Part model, mm, in its own coordinate system. A direction names the side the tool comes from. Round coordinates to 2 decimals unless told otherwise and drop trailing zeros. Loops run counter-clockwise (first coordinate to the right, second up) from the corner with the lowest first, then second, coordinate; pieces in that order, holes last. Notation, with made-up numbers: (-4, 13) - (46, 13) arc R31 cw to (46, 45) - close; hole circle Ø2 at (12, 31.25). An arc over 180 degrees is marked (long way). Put each result on its own line as item: value.
from build123d import *

# Parameters (mm, degrees)
BOSS_EXTRUDE1_DEPTH = 13


with BuildPart() as part:
    # Sketch1 → Boss-Extrude1 (new body)
    with BuildSketch(Plane.XY):
        with BuildLine():
            Line((169.562304459, -46.160309931), (169.552568547, -34.320764913))
            ThreePointArc((169.552568547, -34.320764913), (167.950993273, -32.115534783), (165.631816979, -30.683925688))
            Line((165.631816979, -30.683925688), (164.32472896, -30.359173472))
            ThreePointArc((164.32472896, -30.359173472), (159.414987624, -30.865423823), (155.959571946, -34.389902778))
            Line((155.959571946, -34.389902778), (153.531390597, -39.695181294))
            Line((153.531390597, -39.695181294), (157.716593531, -42.649808935))
            ThreePointArc((157.716593531, -42.649808935), (158.460324124, -45.836019732), (155.520515025, -47.27219413))
            Line((155.520515025, -47.27219413), (152.052832095, -46.502518371))
            add(Edge.make_bspline(
                [(158.254307893, -49.702990605), (156.613856565, -49.334233495), (153.519768391, -49.291899755), (152.26174626, -47.033082798), (152.052832095, -46.502518371)],
                knots=[0, 0, 0, 0, 0.763192253, 1, 1, 1, 1], degree=3))
            Line((158.254307893, -49.702990605), (158.172150747, -49.796885596))
            Line((158.172150747, -49.796885596), (169.562304459, -46.160309931))
        make_face()
    extrude(amount=BOSS_EXTRUDE1_DEPTH)


solid = part.part
1. Band-saw the part on B-B (y = -44). List the corners of the cut face in (x, z).
A:
outline: (158.62, 0) - (169.56, 0) - (169.56, 13) - (158.62, 13) - close
2. Band-saw the part on A-A (x = 159). List the corners of the cut face in (y, z).
A:
outline: (-49.53, 0) - (-31.08, 0) - (-31.08, 13) - (-49.53, 13) - close
3. Pin check, flat tips, straight feed: P1, Ø5, axis at y = -34, z = 9.5, coming from the -X side; P2, Ø3, axis at x = 156.5, z = 2.5, coming from the -Y side; P3, Ø5, axis at y = -35.5, z = 4.5, coming from the -X side; P4, Ø2, axis at x = 156.5, y = -36.5, coming from the -Z side. Stop position of each tip, or through.
A:
P1: stops at x = 154.99
P2: stops at y = -49.65
P3: stops at x = 154.31
P4: stops at z = 0
4. Probe line 1 along Y through (x, z) = (155.25, 5.5); line 2 along Y through (x, z) = (155.5, 1.75); line 3 along X through (y, z) = (-42.75, 5.75). List the from-to ranges inside material, lowest first. Write a range as [from, to].
A:
line 1: y = [-49.14, -47.21], [-40.91, -35.94]
line 2: y = [-49.2, -47.27], [-41.08, -35.39]
line 3: x = [157.84, 169.56]
5. Two-plate mould, pull along X, no slides. Class faces 1 (the flat face through (163.8, -48, 6.4)), 2 (the flat face through (153.811, -46.893, 6.409)), 3 (the cylindrical face through (158.48, -45.79, 6.41)), 4 (the cylindrical face through (159.479, -30.835, 6.409)): pulls with the +X half, pulls with the -X half, needs draft (parallel to the pull), parting line crosses it, or undercut.
A:
face 1: pulls with the +X half
face 2: undercut
face 3: undercut
face 4: parting line crosses it
6. Tool access for faces 5 (the flat face through (154.76, -37.01, 6.41)), 6 (the flat face through (155.59, -41.15, 6.41)): list every direction of +Z, -Z, +X, -X, +Y, -Y with a clear straight run to the whole face (end or side of a thin tool).
A:
face 5: +Z, -Z, -X, +Y
face 6: +Z, -Z, -X
